The drawing under review shows one solid part. Ordinate dimensions are in mm from its lowest x, y, z. Coordinates: 2 decimals unless noted, no trailing zeros. Write each loop counter-clockwise with the first axis right and the second up, starting at its lowest first coordinate (ties: lowest second). Pieces come first, ordered by that corner, then holes. Notation, with made-up numbers: (72.25, -32) - (87.25, -32) arc R31 cw to (87.25, -8) - close; hole circle Ø4 at (25.5, 3). An arc over 180 degrees is marked (long way). Put each result on its own line as item: value. Start each with the question number.
Item 1: Consider section B-B on x = 148.5. Give the boundary of the cut face in (y, z) (1 decimal).
Item 2: To check wall thickness, follow L1, parallel to X at y = 0.65, z = 26.5 (1 decimal); L2, parallel to Z at x = 148.5, y = 1.3 (1 decimal). State the ranges of each line that lie inside material, in increasing order. Write a range as [from, to].
Item 3: Consider section A-A on z = 26.5. Give the boundary of the cut face in (x, y) (1 decimal).
Item 4: For pin 1 (1.5 mm diameter, centred on y = 1.5, z = 86.5, fed in from -X), flat-tipped, find the tip position at first contact; note if it passes through.
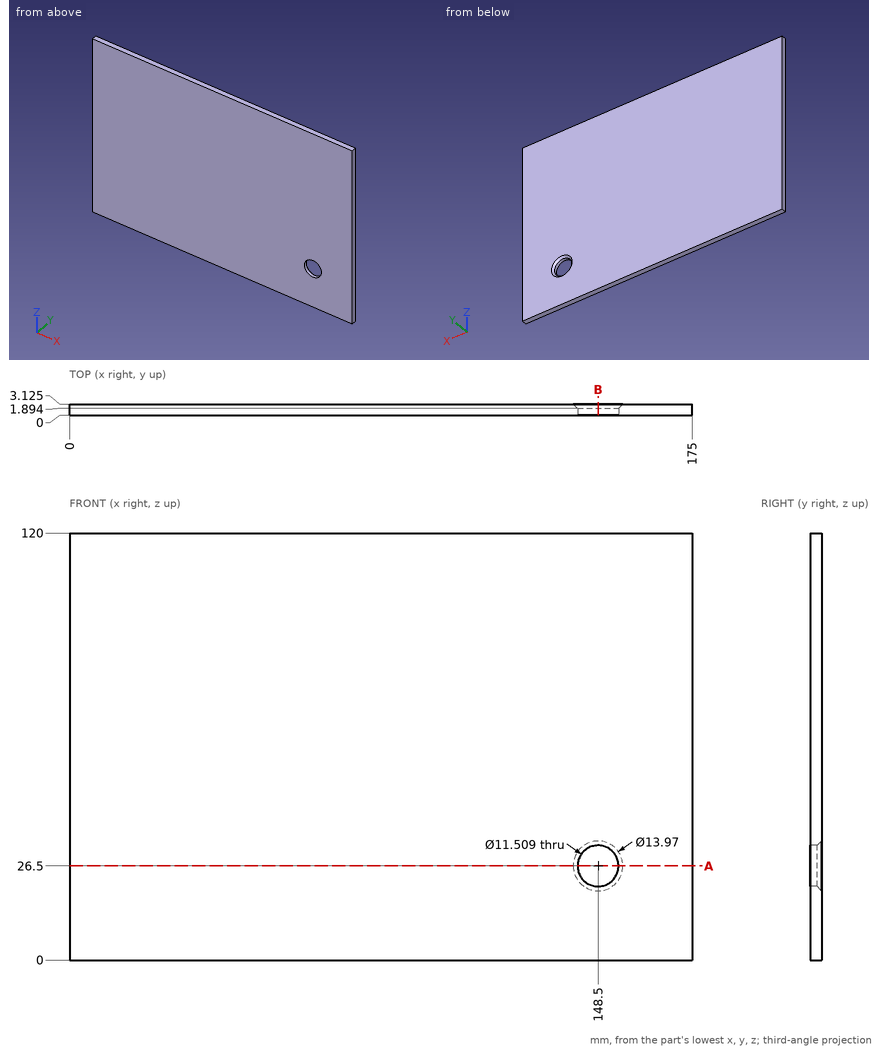
Report:
1. outline: (0, 0) - (3.1, 0) - (3.1, 19.5) - (1.9, 20.7) - (0, 20.7) - close; (0, 32.3) - (1.9, 32.3) - (3.1, 33.5) - (3.1, 120) - (0, 120) - close
2. L1: [0, 142.7], [154.3, 175]
2. L2: [0, 20.7], [32.3, 120]
3. outline: (0, 0) - (142.7, 0) - (142.7, 1.9) - (141.5, 3.1) - (0, 3.1) - close; (154.3, 0) - (175, 0) - (175, 3.1) - (155.5, 3.1) - (154.3, 1.9) - close
4. pin 1: x = 0
